For this review, take the finished solid that the model builds, in its own axes (mm). A direction names the side the tool comes from. Round coordinates to 2 decimals unless told otherwise and drop trailing zeros. Loops run counter-clockwise (first coordinate to the right, second up) from the corner with the lowest first, then second, coordinate; pieces in that order, holes last.
1) Mouldability with a two-part tool opening along X and no side actions: class faces 1 (the flat face through (5, 9.525, -5)), 2 (the cylindrical face through (8.65, 5.71, -8.96)), 3 (the flat face through (4, 1.191, -2)) as pulls with the +X half, pulls with the -X half, needs draft (parallel to the pull), parting line crosses it, or undercut.
2) Take a section at A-A (y = 4.5). State the section outline as (x, z) points, then the cut area to 3 significant figures.
3) Take a section at B-B (y = 10). State the section outline as (x, z) points (1 decimal).
4) Wall thickness on L1, parallel to Z at x = 5.25, y = 6.5; L2, parallel to Z at x = 7, y = 1.75; L3, parallel to X at y = 2.25, z = -5.5: over which ranges is each line inside the solid? List them lowest first.
5) Tool access review of faces 4 (the cylindrical face through (7.27, 4.3, -4.06)), 5 (the flat face through (7, 11.906, -5)), 6 (the cylindrical face through (4.551, 10.732, -3.693)): name each direction out of +Z, -Z, +X, -X, +Y, -Y from which nothing blocks a thin tool from reaching the whole face with its end or side.
6) Insertion check: pin 1 (1 mm diameter, centred on x = 8.5, z = -6, fed in from +Y); pin 2 (3.5 mm diameter, centred on x = 5.16, z = -5.16, fed in from -Y); pin 3 (3 mm diameter, centred on x = 3, y = 7, fed in from -Z). Each pin has a flat end and moves straight along its axis. Give the tip position at first contact, or say it passes through.
```python
from build123d import *

# Parameters (mm, degrees)
SKETCH2_R           = 5.159375
BOSS_EXTRUDE2_DEPTH = 11.90625
CUT_EXTRUDE1_START  = -1.5875
SKETCH3_R           = 5.159375
SKETCH3_R_2         = 2.38125
CUT_EXTRUDE1_DEPTH  = 1.5875
SKETCH4_R           = 5.159375
SKETCH4_R_2         = 3.175
CUT_EXTRUDE2_DEPTH  = 1.190625
SKETCH5_R           = 2.38125
CUT_EXTRUDE3_DEPTH  = 8.73125
SKETCH6_R           = 1.5875
CUT_EXTRUDE4_DEPTH  = 2.38125
FILLET1_R           = 1.5875
FILLET3_R           = 0.1016


with BuildPart() as part:
    # Sketch2 → Boss-Extrude2 (new body)
    with BuildSketch(Plane(origin=(0, 0, 0), x_dir=(1, 0, 0), z_dir=(0, 1, 0))):
        with Locations(Location((5.159375, 5.159375, 0), (0, 0, 270))):
            Circle(SKETCH2_R)
    extrude(amount=BOSS_EXTRUDE2_DEPTH)

    # Sketch3 → Cut-Extrude1 (cut)
    with BuildSketch(Plane(origin=(0, 11.90625, 0), x_dir=(1, 0, 0), z_dir=(0, 1, 0)).offset(CUT_EXTRUDE1_START)):
        with Locations(Location((5.159375, 5.159375, 0), (0, 0, 270))):
            Circle(SKETCH3_R)
        with Locations(Location((5.159375, 5.159375, 0), (0, 0, 270))):
            Circle(SKETCH3_R_2, mode=Mode.SUBTRACT)
    extrude(amount=CUT_EXTRUDE1_DEPTH, mode=Mode.SUBTRACT)

    # Sketch4 → Cut-Extrude2 (cut)
    with BuildSketch(Plane.XZ):
        with Locations(Location((5.159375, -5.159375, 0), (0, 0, 270))):
            Circle(SKETCH4_R)
        with Locations(Location((5.159375, -5.159375, 0), (0, 0, 270))):
            Circle(SKETCH4_R_2, mode=Mode.SUBTRACT)
    extrude(amount=-CUT_EXTRUDE2_DEPTH, mode=Mode.SUBTRACT)

    # Sketch5 → Cut-Extrude3 (cut)
    with BuildSketch(Plane.XZ):
        with Locations(Location((5.159375, -5.159375, 0), (0, 0, 90))):
            Circle(SKETCH5_R)
    extrude(amount=-CUT_EXTRUDE3_DEPTH, mode=Mode.SUBTRACT)

    # Sketch6 → Cut-Extrude4 (cut)
    with BuildSketch(Plane(origin=(0, 11.90625, 0), x_dir=(1, 0, 0), z_dir=(0, 1, 0))):
        with Locations(Location((5.159375, 5.159375, 0), (0, 0, 270))):
            Circle(SKETCH6_R)
    extrude(amount=-CUT_EXTRUDE4_DEPTH, mode=Mode.SUBTRACT)

    # Fillet1
    fillet1_edges = [part.edges().sort_by_distance(p)[0] for p in [
        (5.159375, 1.190625, -10.31875),
        (5.159375, 10.31875, -10.31875),
    ]]
    fillet(fillet1_edges, radius=FILLET1_R)

    # Fillet3
    fillet3_edges = [part.edges().sort_by_distance(p)[0] for p in [
        (5.159375, 11.90625, -7.540625),
    ]]
    fillet(fillet3_edges, radius=FILLET3_R)


solid = part.part
```
Response:
1. face 1: undercut
1. face 2: parting line crosses it
1. face 3: needs draft
2. outline: circle Ø10.32 at (5.16, -5.16); hole circle Ø4.76 at (5.16, -5.16)
2. area: 65.8 mm2
3. outline: circle Ø9.1 at (5.2, -5.2); hole circle Ø3.2 at (5.2, -5.2)
4. L1: z = -10.32 to -7.54, -2.78 to 0
4. L2: z = -9.57 to -6.67, -3.65 to -0.75
4. L3: x = 0.1 to 2.8, 7.52 to 10.22
5. face 4: -Y
5. face 5: +Z, -Z, +X, -X, +Y
5. face 6: +Y
6. pin 1: stops at y = 10.32
6. pin 2: stops at y = 8.73
6. pin 3: stops at z = -10.28
